```python
from build123d import *

# Parameters (mm, degrees)
SKETCH1_R           = 63.5
BOSS_EXTRUDE1_DEPTH = 6.35
SKETCH2_R           = 57.15
SKETCH2_R_2         = 50.8
CUT_EXTRUDE1_DEPTH  = 1.27
SKETCH4_R           = 1.190625
CUT_EXTRUDE2_DEPTH  = 91.02678768
SKETCH5_R           = 1.5875
CUT_EXTRUDE3_DEPTH  = 1.27
SKETCH6_R           = 5.55625
CUT_EXTRUDE4_DEPTH  = 91.02678768


with BuildPart() as part:
    # Sketch1 → Boss-Extrude1 (new body)
    with BuildSketch(Plane.XY):
        Circle(SKETCH1_R)
    extrude(amount=BOSS_EXTRUDE1_DEPTH)

    # Sketch2 → Cut-Extrude1 (cut)
    with BuildSketch(Plane(origin=(0, 0, 0), x_dir=(-1, 0, 0), z_dir=(0, 0, -1))):
        Circle(SKETCH2_R)
        Circle(SKETCH2_R_2, mode=Mode.SUBTRACT)
    extrude(amount=-CUT_EXTRUDE1_DEPTH, mode=Mode.SUBTRACT)

    # Sketch4 → Cut-Extrude2 (cut, through all)
    with BuildSketch(Plane(origin=(0, 0, 0), x_dir=(-1, 0, 0), z_dir=(0, 0, -1))):
        with Locations((0, 60.96)):
            Circle(SKETCH4_R)
        with Locations((60.96, 0)):
            Circle(SKETCH4_R)
        with Locations((0, -60.96)):
            Circle(SKETCH4_R)
        with Locations((-60.96, 0)):
            Circle(SKETCH4_R)
    extrude(amount=-CUT_EXTRUDE2_DEPTH, mode=Mode.SUBTRACT)

    # Sketch5 → Cut-Extrude3 (cut)
    with BuildSketch(Plane.XY.offset(6.35)):
        with Locations((0, 60.96)):
            Circle(SKETCH5_R)
        with Locations((60.96, 0)):
            Circle(SKETCH5_R)
        with Locations((0, -60.96)):
            Circle(SKETCH5_R)
        with Locations((-60.96, 0)):
            Circle(SKETCH5_R)
    extrude(amount=-CUT_EXTRUDE3_DEPTH, mode=Mode.SUBTRACT)

    # Sketch6 → Cut-Extrude4 (cut, through all)
    with BuildSketch(Plane(origin=(0, 0, 0), x_dir=(-1, 0, 0), z_dir=(0, 0, -1))):
        Circle(SKETCH6_R)
    extrude(amount=-CUT_EXTRUDE4_DEPTH, mode=Mode.SUBTRACT)


solid = part.part
```
The listing builds one solid part. Answer for the finished solid, in the listing's coordinates (mm). A direction names the side the tool comes from. Give positions to 0.01 mm unless a question says otherwise; leave off trailing zeros. Loops run counter-clockwise (first coordinate to the right, second up) from the corner with the lowest first, then second, coordinate; pieces in that order, holes last. Notation, with made-up numbers: (11, 72) - (57, 72) arc R21 ccw to (57, 89) - close; hole circle Ø11 at (-4.5, 25.5). An arc over 180 degrees is marked (long way). Return JSON: item names as keys, results as strings. Group by question number.
1. Find section B-B (x = -53). Write down the section's boundary in (y, z) (3 decimals).
2. Find section C-C (y = -23.5). Write down the section's boundary in (x, z).
3. Given pin 1 Ø3 at (x, y) = (0, 60.96) entering from -Z; pin 2 Ø3 at (y, z) = (48.5, 4.5) entering from -X; pin 3 Ø3 at (y, z) = (10, 1.5) entering from -X; pin 4 Ø3 at (y, z) = (35.5, 2) entering from -X, each flat-ended and moving along its own axis, determine where each tip first touches the part or whether it passes through.
4. Determine the mould class of faces 1 (the flat face through (-60, 1, 5.08)), 2 (the cylindrical face through (-13.77, -61.99, 3.13)), 3 (the flat face through (-47, -33, 0)) for opening direction Y: pulls with the +Y half, pulls with the -Y half, needs draft (parallel to the pull), parting line crosses it, or undercut.
5. Find section A-A (z = 2.5). Write down the section's boundary in (x, y), then the cut area to 3 significant figures.
6. Straight lines are drawn through the part: line 1 (Y direction, x = 0, z = 3.3); line 2 (Y direction, x = 0, z = 5.95); line 3 (Y direction, x = 37, z = 1). For each, find the intervals that lie inside material, in ascending order. Write a range as [from, to].
7. Which of the six approach directions +Z, -Z, +X, -X, +Y, -Y give full straight-line access (tool end or side, diameter ignored) to faces 4 (the flat face through (11, 1, 0)), 5 (the cylindrical face through (11.012, -49.592, 0.626)), 6 (the cylindrical face through (-0.207, -59.386, 5.724))?
8. Find section D-D (y = 24). Write down the section's boundary in (x, z).
Verdict:
{
 "1": {"outline": "(-34.975, 0) - (-21.38, 0) - (-21.38, 1.27) - (21.38, 1.27) - (21.38, 0) - (34.975, 0) - (34.975, 6.35) - (-34.975, 6.35) - close"},
 "2": {"outline": "(-58.99, 0) - (-52.09, 0) - (-52.09, 1.27) - (-45.04, 1.27) - (-45.04, 0) - (45.04, 0) - (45.04, 1.27) - (52.09, 1.27) - (52.09, 0) - (58.99, 0) - (58.99, 6.35) - (-58.99, 6.35) - close"},
 "3": {"pin 1": "stops at z = 0", "pin 2": "stops at x = -42.7", "pin 3": "stops at x = -62.93", "pin 4": "stops at x = -53.63"},
 "4": {"face 1": "undercut", "face 2": "parting line crosses it", "face 3": "needs draft"},
 "5": {"outline": "circle Ø127 at (0, 0); hole circle Ø2.38 at (-60.96, 0); hole circle Ø11.11 at (0, 0); hole circle Ø2.38 at (0, -60.96); hole circle Ø2.38 at (0, 60.96); hole circle Ø2.38 at (60.96, 0)", "area": "12,600 mm^2"},
 "6": {"line 1": "y = [-63.5, -62.15], [-59.77, -5.56], [5.56, 59.77], [62.15, 63.5]", "line 2": "y = [-63.5, -62.55], [-59.37, -5.56], [5.56, 59.37], [62.55, 63.5]", "line 3": "y = [-51.61, -43.56], [-34.81, 34.81], [43.56, 51.61]"},
 "7": {"face 4": "-Z, +X, -X, +Y, -Y", "face 5": "-Z", "face 6": "+Z"},
 "8": {"outline": "(-58.79, 0) - (-51.87, 0) - (-51.87, 1.27) - (-44.77, 1.27) - (-44.77, 0) - (44.77, 0) - (44.77, 1.27) - (51.87, 1.27) - (51.87, 0) - (58.79, 0) - (58.79, 6.35) - (-58.79, 6.35) - close"}
}
